```python
from build123d import *

# Parameters (mm, degrees)
CYLINDER002_R     = 20
CYLINDER002_DEPTH = 20
CYLINDER001_W     = 30
CYLINDER001_H     = 10
CYLINDER001_ANGLE = 23
ARRAY_COUNT       = 8
CYLINDER_R        = 30
CYLINDER_DEPTH    = 90


with BuildPart() as cylinder002:
    # Cylinder002 → Cylinder002 (new body)
    with BuildSketch(Plane.XY.offset(70)):
        Circle(CYLINDER002_R)
    extrude(amount=CYLINDER002_DEPTH)


with BuildPart() as array:
    # Cylinder001 → Cylinder001 (revolve)
    with BuildSketch(Plane(origin=(0, 0, 80), x_dir=(1, 0, 0), z_dir=(0, -1, 0))):
        with Locations((15, 5)):
            Rectangle(CYLINDER001_W, CYLINDER001_H)
    revolve(axis=Axis((0, 0, 80), (0, 0, 1)), revolution_arc=CYLINDER001_ANGLE)

    # Array: Array ×8 about axis
    array_axis = Axis((0, 0, 0), (0, 0, 1))


with BuildPart() as array_1:
    add(array.part)
    for i in range(1, ARRAY_COUNT):
        add(array.part.rotate(array_axis, i * 360 / ARRAY_COUNT))


with BuildPart() as cut001:
    # Cylinder → Cylinder (new body)
    with BuildSketch(Plane.XY):
        Circle(CYLINDER_R)
    extrude(amount=CYLINDER_DEPTH)

    # Cut: cut Array
    add(array_1.part, mode=Mode.SUBTRACT)

    # Cut001: cut Cylinder002
    add(cylinder002.part, mode=Mode.SUBTRACT)


solid = cut001.part
```
For this review, take the finished solid that the model builds, in its own axes (mm). A direction names the side the tool comes from. Give positions to 0.01 mm unless a question says otherwise; leave off trailing zeros. Write each loop counter-clockwise with the first axis right and the second up, starting at its lowest first coordinate (ties: lowest second). Pieces come first, ordered by that corner, then holes. Notation, with made-up numbers: M 76.25,47 L 121.25,47 A10 ccw 121.25,57 Z; hole C 50.5,55 d10. An arc over 180 degrees is marked long. Answer as CSV lines item,"result".
1. Consider section C-C, the plane z = 14. Write out the cut boundary in (x, y), then the cut area to 3 significant figures.
Findings:
outline,"C 0,0 d60"
area,"2,830 mm2"
2. Consider section B-B, the plane x = -3. Write out the cut boundary in (y, z), then the cut area to 3 significant figures.
Findings:
outline,"M -29.85,0 L 29.85,0 L 29.85,80 L 19.77,80 L 19.77,70 L -19.77,70 L -19.77,90 L -29.85,90 Z"
area,"4,480 mm2"
3. Consider section A-A, the plane y = -23. Write out the cut boundary in (x, z), then the cut area to 3 significant figures.
Findings:
outline,"M -19.26,0 L 19.26,0 L 19.26,90 L 9.76,90 L 9.76,80 L 0,80 L 0,90 L -9.29,90 L -9.29,80 L -19.26,80 Z"
area,"3,270 mm2"
4. Wall thickness on line 1 (Y direction, x = 0, z = 76.5); line 2 (X direction, y = -5, z = 70.5); line 3 (Z direction, x = 8, y = 1): over which ranges is each line inside the solid? List them lowest first.
Findings:
line 1,"y = -30 to -20, 20 to 30"
line 2,"x = -29.58 to -19.36, 19.36 to 29.58"
line 3,"z = 0 to 70"
5. For faces 1 (the flat face through (24, 5, 80)), 2 (the flat face through (20, -14, 80)), 3 (the flat face through (0, 25, 85)), 4 (the flat face through (5, -24, 80)), 5 (the flat face through (-22.95, -9.74, 85.07)), list the 3-axis set-ups (+Z, -Z, +X, -X, +Y, -Y) from which the entire face can be reached by the end or side of a thin tool; tool diameter is ignored.
Findings:
face 1,"+Z, +X"
face 2,"+Z"
face 3,"+Z, +Y"
face 4,"+Z, -Y"
face 5,"+Z, -X"
6. For pin 1 (8 mm diameter, centred on y = -19, z = 15.5, fed in from -X); pin 2 (4 mm diameter, centred on x = 12, z = 43, fed in from -Y); pin 3 (4 mm diameter, centred on x = -16, y = -22.5, fed in from +Z), all flat-tipped, find the tip position at first contact; note any pin that passes through.
Findings:
pin 1,"stops at x = -25.98"
pin 2,"stops at y = -28.28"
pin 3,"stops at z = 80"
7. Consider section D-D, the plane y = -5. Write out the cut boundary in (x, z).
Findings:
outline,"M -29.58,0 L 29.58,0 L 29.58,90 L 19.36,90 L 19.36,70 L -19.36,70 L -19.36,80 L -29.58,80 Z"
8. Draft analysis for pull direction Y (two halves, no side actions). For faces 6 (the flat face through (-9.74, 22.95, 85.07)), 7 (the flat face through (-24, -5, 80)), 8 (the flat face through (24, -4, 90)), state which applies: +Y half, -Y half, draft (parallel to the pull), parting line (faces both ways), or undercut.
Findings:
face 6,"+Y half"
face 7,"undercut"
face 8,"draft"
